Geometry: final body of the model. Coordinates: model frame, mm. Coordinates: 2 decimals unless noted, no trailing zeros. Loops run counter-clockwise (first coordinate to the right, second up) from the corner with the lowest first, then second, coordinate; pieces in that order, holes last. Notation, with made-up numbers: (1.25, 14.25) - (27.25, 14.25) arc R12 cw to (27.25, 22.25) - close; hole circle Ø9 at (73.5, -16.5). An arc over 180 degrees is marked (long way). Put each result on its own line as item: value. Start each with the question number.
1) Material intervals for line 1 along Z through (x, y) = (12, 0.4); line 2 along X through (y, z) = (1.55, 96.5); line 3 along X through (y, z) = (1.4, -14.5), sorted ascending. Write a range as from..to.
2) Contact query for flat-ended pins moving along their axis: pin 1 Ø1.8 at (x, z) = (0, 10) entering from -Y; pin 2 Ø1 at (y, z) = (1, -8) entering from -X; pin 3 Ø1 at (x, y) = (71, 1.5) entering from +Z. Output: stop coordinate, or through.
3) Section B-B on y = 1.45. Output: boundary loops of the cut face in (x, z).
4) Section D-D on x = 41. Output: boundary loops of the cut face in (y, z).
5) Section A-A on x = 12. Output: boundary loops of the cut face in (y, z), and give its area (3 significant figures).
6) Section C-C on z = 80. Output: boundary loops of the cut face in (x, y), and give its area (3 significant figures).
Autodesk Inventor part; units mm, degrees
ref_plane "YZ Plane" through (0, 0, 0) normal (1, 0, 0) x (0, 1, 0)
ref_plane "XZ Plane" through (0, 0, 0) normal (0, 1, 0) x (-1, 0, 0)
ref_plane "XY Plane" through (0, 0, 0) normal (0, 0, 1) x (1, 0, 0)
sketch "Sketch1" plane through (0, 0, 0) normal (0, 1, 0) x (-1, 0, 0)
  line L0 (0, 0) -> (0, -25)
  line L1 (0, 0) -> (25, 0)
  line L2 (0, 0) -> (-107.2462, 89.9903)
  line L3 (0, 0) -> (140, 0) construction
  line L4 (-107.2462, 89.9903) -> (-102.7467, 95.3526)
  line L5 (-102.7467, 95.3526) -> (-110.9666, 84.0198)
  line L6 (-107.2462, 89.9903) -> (-114.9067, 96.4181)
  line L7 (-114.9067, 96.4181) -> (-120.6117, 88.2052)
  line L8 (-120.6117, 88.2052) -> (-109.2017, 104.6311)
  circle A0 centre (-109.2017, 104.6311) radius 1.5
  circle A1 centre (-102.7467, 95.3526) radius 1.5
  circle A2 centre (-110.9666, 84.0198) radius 1.5
  circle A3 centre (-120.6117, 88.2052) radius 1.5
  circle A4 centre (-111.0764, 93.2042) radius 15
  arc A5 (25, 0) -> (-19.1511, 16.0697) centre (0, 0) ccw
  arc A6 (-18.4671, 16.8513) -> (0, -25) centre (0, 0) ccw
  line L9 (-102.25, 105.3325) -> (14.7107, 20.2138)
  line L10 (-121.4878, 82.4058) -> (-17.3522, -17.9973)
  dimension "d0" = 25
  dimension "d1" = 25
  dimension "d2" = 140
  dimension "d3" = 140
  dimension "d4" = 7
  dimension "d5" = 14
  dimension "d6" = 10
  dimension "d7" = 10
  dimension "d8" = 20
  dimension "d9" = 3
  dimension "d10" = 3
  dimension "d11" = 3
  dimension "d12" = 3
  dimension "d13" = 30
extrude "Extrusion1" add sketch "Sketch1" along normal blind 2 contours L2 A5 L1 | L0 A6 L2 | A6 L10 A4 L2 | L2 A4 L9 A5 | L2 L4 A1 L5 | A4
sketch "Sketch2" plane through (0, 2, 0) normal (0, 1, 0) x (1, 0, 0)
  line L0 (0, 25) -> (0, 0)
  line L1 (0, 25) -> (0, 14)
  line L2 (0, 14) -> (12, 14)
  circle A0 centre (12, 14) radius 2
  line L3 (0, 25) -> (0, 0)
  line L4 (0, 0) -> (-10.922, 0)
  line L5 (0, 0) -> (-25, 0)
  line L6 (-10.922, 0) -> (-10.922, -12)
  circle A1 centre (-10.922, -12) radius 2
  dimension "d16" = 11
  dimension "d17" = 12
  dimension "d18" = 4
  dimension "d24" = 10.922
  dimension "d25" = 12
  dimension "d26" = 4
extrude "Extrusion2" cut sketch "Sketch2" against normal blind 2 contours A0
extrude "Extrusion3" cut sketch "Sketch2" against normal blind 2 contours A1
sketch "Sketch3" plane through (0, 2, 0) normal (0, 1, 0) x (1, 0, 0)
  line L0 (0, 25) -> (0, 0)
  line L1 (0, 0) -> (0, -10)
  circle A0 centre (0, -10) radius 1.5
  dimension "d29" = 10
  dimension "d30" = 3
extrude "Extrusion4" cut sketch "Sketch3" against normal blind 2
properties part number "arm"
Answer block:
1. line 1: z = -21.93..-16, -12..39.65
1. line 2: x = 90.11..101.78, 103.71..125.71
1. line 3: x = 0..10.06, 13.94..20.98
2. pin 1: passes through
2. pin 2: stops at x = 0
2. pin 3: stops at z = 82.95
3. outline: (-25, 0) - (0, 0) - (0, -25) arc R25 ccw to (17.35, -18) - (121.49, 82.41) arc R15 ccw to (102.25, 105.33) - (-14.71, 20.21) arc R25 ccw to start; hole circle Ø4 at (-10.92, 12); hole circle Ø3 at (0, 10); hole circle Ø4 at (12, -14); hole circle Ø3 at (102.75, 95.35); hole circle Ø3 at (109.2, 104.63); hole circle Ø3 at (110.97, 84.02); hole circle Ø3 at (120.61, 88.21)
4. outline: (0, 4.8) - (2, 4.8) - (2, 60.76) - (0, 60.76) - close
5. outline: (0, -21.93) - (2, -21.93) - (2, -16) - (0, -16) - close; (0, -12) - (2, -12) - (2, 39.65) - (0, 39.65) - close
5. area: 115 mm²
6. outline: (67.44, 0) - (118.99, 0) - (118.99, 2) - (67.44, 2) - close
6. area: 103 mm²
